Read the model definition and answer for the solid it produces. Units are mm, in the model's axes. A direction names the side the tool comes from. Coordinates: 2 decimals unless noted, no trailing zeros. Write each loop counter-clockwise with the first axis right and the second up, starting at its lowest first coordinate (ties: lowest second). Pieces come first, ordered by that corner, then holes. Notation, with made-up numbers: M -16,48 L 13,48 A30 cw 13,72 Z; hole C 64.5,63.5 d4. An arc over 180 degrees is marked long. Write item = value, one per line.
from build123d import *

# Parameters (mm, degrees)
F0_R     = 24.25
F0_R_2   = 3.625
F1_DEPTH = 4
F2_R     = 7.5
F2_R_2   = 3.625
F3_DEPTH = 4.75
F4_R     = 2.020962
F5_DEPTH = 4.001
F6_R     = 2.5


with BuildPart() as f1:
    # F0 (on Top) → F1 (new body)
    with BuildSketch(Plane.XY):
        Circle(F0_R)
        with BuildLine():
            Line((8.950036, 4.46059), (8.950036, 13.225189))
            ThreePointArc((8.950036, 13.225189), (10.098851, 15.035019), (12.22552, 14.765688))
            ThreePointArc((12.22552, 14.765688), (19.163787, -0.488041), (11.458089, -15.368835))
            ThreePointArc((11.458089, -15.368835), (9.299885, -15.51842), (8.268192, -13.616887))
            Line((8.268192, -13.616887), (8.950036, -4.46059))
            ThreePointArc((8.950036, -4.46059), (10, 0), (8.950036, 4.46059))
        make_face(mode=Mode.SUBTRACT)
        with BuildLine():
            Line((-8.268192, 13.616887), (-8.950036, 4.46059))
            ThreePointArc((-8.950036, 4.46059), (-10, 0), (-8.950036, -4.46059))
            Line((-8.950036, -4.46059), (-8.950036, -13.225189))
            ThreePointArc((-8.950036, -13.225189), (-10.098851, -15.035019), (-12.22552, -14.765688))
            ThreePointArc((-12.22552, -14.765688), (-19.163787, 0.488041), (-11.458089, 15.368835))
            ThreePointArc((-11.458089, 15.368835), (-9.299885, 15.51842), (-8.268192, 13.616887))
        make_face(mode=Mode.SUBTRACT)
        Circle(F0_R_2, mode=Mode.SUBTRACT)
    extrude(amount=F1_DEPTH)

    # F2 (on face) → F3 (join)
    with BuildSketch(Plane.XY.offset(4)):
        Circle(F2_R)
        Circle(F2_R_2, mode=Mode.SUBTRACT)
    extrude(amount=F3_DEPTH)

    # F4 (on face) → F5 (cut, through all)
    with BuildSketch(Plane.XY.offset(4)):
        Polygon((-5.234685, 11.362989), (0, 11.362989), (0, 17.41166), align=None)
        Polygon((0, 17.41166), (0, 11.362989), (5.234685, 11.362989), align=None)
        Polygon((0, -11.362989), (-5.234685, -11.362989), (0, -17.41166), (5.234685, -11.362989), align=None)
        with Locations((0, 20.410169)):
            Circle(F4_R)
        with Locations((0, -20.410169)):
            Circle(F4_R)
    extrude(amount=-F5_DEPTH, mode=Mode.SUBTRACT)

    # F6 (on Front) → F7 (revolve, cut)
    with BuildSketch(Plane.XZ):
        with Locations((-25.767528, 2.014234)):
            Circle(F6_R)
    revolve(axis=Axis((0, 0, 7.021954), (0, 0, -1)), mode=Mode.SUBTRACT)


solid = f1.part
Item 1: Consider line 1 along X through (y, z) = (8.5, 1.75); line 2 along Y through (x, z) = (0, 6.5) (3 decimals); line 3 along X through (y, z) = (-14.5, 1.75). Determine where each line is inside the solid, lowest interval first. Write a range as from..to.
Worked answers:
line_1 = -21.67..-17.18, -8.65..8.95, 17.18..21.67
line_2 = -7.5..-3.625, 3.625..7.5
line_3 = -18.21..-12.54, -9.41..-2.52, 2.52..8.4, 12.54..18.21
Item 2: Find section A-A (y = 0). State how many separate pieces and enclosed holes the cut face has, and give its area (3 significant figures).
Worked answers:
separate_pieces = 4
enclosed_holes = 0
area = 123 mm²
Item 3: Flat-ended cylindrical pins translate along their axes: pin 1 (1.2 mm diameter, centred on x = 0, z = 2.5, fed in from -Y); pin 2 (2.5 mm diameter, centred on x = 0, y = 20.41, fed in from -Z); pin 3 (1.5 mm diameter, centred on x = -1, z = 6.5, fed in from +Y); pin 4 (1.2 mm diameter, centred on y = -11, z = 2, fed in from -X). Find the tip coordinate at first contact, or state that the pin passes through.
Worked answers:
pin_1 = -23.52
pin_2 = through
pin_3 = 7.5
pin_4 = -20.81
Item 4: Which of the six approach directions +Z, -Z, +X, -X, +Y, -Y give full straight-line access (tool end or side, diameter ignored) to faces 4 (the face through (-2.58, 14.43, 2.03)), 5 (the face through (0, -5, 0))?
Worked answers:
face_4 = +Z, -Z
face_5 = -Z, +X, -X, +Y, -Y
Item 5: For a pull along Y with two mould halves and no side action, classify faces 1 (the face through (1.56, 3.44, 8.75)), 2 (the face through (-2.654, -14.345, 2.028)), 3 (the face through (0, 11.363, 2)) as released by +Y, released by -Y, zero draft, split by the parting line, or undercut.
Worked answers:
face_1 = zero draft
face_2 = undercut
face_3 = undercut
Item 6: Find section B-B (z = 6.5). Determine the outline of the cut face in (x, y) (3 decimals).
Worked answers:
outline = C 0,0 d15; hole C 0,0 d7.25
